Source: three-view drawing plus pictorial views. Frame: mm from the lowest corner of the part. A direction names the side the tool comes from. Round coordinates to 2 decimals unless told otherwise and drop trailing zeros. Write each loop counter-clockwise with the first axis right and the second up, starting at its lowest first coordinate (ties: lowest second). Pieces come first, ordered by that corner, then holes. Notation, with made-up numbers: (-16.5, 8.5) - (12.5, 8.5) arc R13 cw to (12.5, 16.5) - close; hole circle Ø1 at (79, 16). An arc over 180 degrees is marked (long way). Write each question's results on one line, items separated by ' | '.
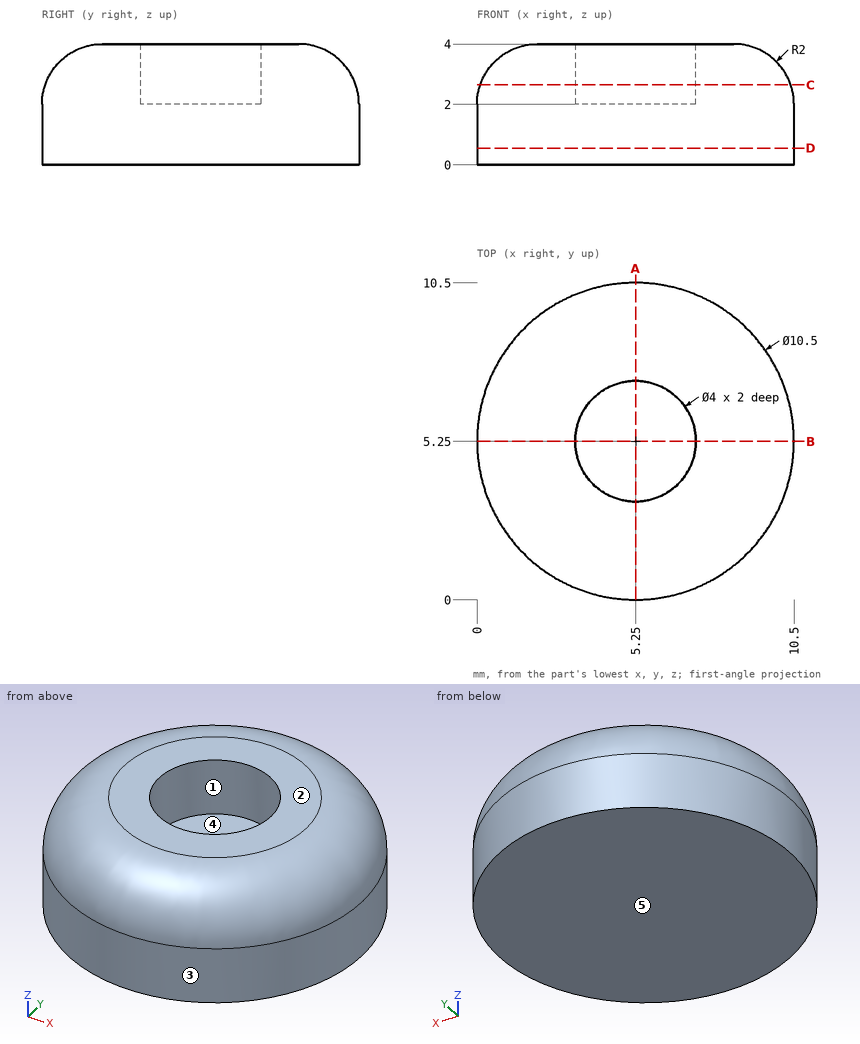
Q1. Section query A-A, the plane x = 5.25. Return loops of the section in (y, z), plus the area to 3 significant figures.
Answer block:
outline: (0, 0) - (10.5, 0) - (10.5, 2) arc R2 ccw to (8.5, 4) - (7.25, 4) - (7.25, 2) - (3.25, 2) - (3.25, 4) - (2, 4) arc R2 ccw to (0, 2) - close | area: 32.3 mm2
Q2. Section query C-C, the plane z = 2.65. Return loops of the section in (x, y), plus the area to 3 significant figures.
Answer block:
outline: circle Ø10.28 at (5.25, 5.25); hole circle Ø4 at (5.25, 5.25) | area: 70.5 mm2
Q3. Mould query, pull axis Y, two halves, no side actions, for the marked faces 3, 4 and 5. Classes: pulls with the +Y half, pulls with the -Y half, needs draft (parallel to the pull), parting line crosses it, or undercut.
Answer block:
face 3: parting line crosses it | face 4: undercut | face 5: needs draft
Q4. Section query D-D, the plane z = 0.55. Return loops of the section in (x, y).
Answer block:
outline: circle Ø10.5 at (5.25, 5.25)
Q5. Access query for the marked faces 1 and 2. Directions: +Z, -Z, +X, -X, +Y, -Y. A direction counts if a zero-diameter tool reaches every point of the face in a straight line with its end or side. Return the directions, or none.
Answer block:
face 1: +Z | face 2: +Z, +X, -X, +Y, -Y
Q6. Pin query (flat end, axial travel): pin 1 (1.2 mm diameter, centred on x = 5, y = 5, fed in from +Z); pin 2 (1.5 mm diameter, centred on x = 5, z = 3, fed in from +Y); pin 3 (2 mm diameter, centred on x = 3.5, z = 3, fed in from -Y). Return the tip coordinate at first contact, or that it passes through.
Answer block:
pin 1: z = 2 | pin 2: y = 10.48 | pin 3: y = 0.13
Q7. Ray query, line 1 along Z through (x, y) = (4, 4); line 2 along Y through (x, z) = (5.25, 2.6); line 3 along Y through (x, z) = (5.5, 3.1). Return the intervals inside material, ascending.
Answer block:
line 1: 0 to 2 | line 2: 0.09 to 3.25, 7.25 to 10.41 | line 3: 0.34 to 3.27, 7.23 to 10.16
